Input: part model. Units: mm. Frame: model coordinates. Face numbers are marked on the shaded views. A direction names the side the tool comes from. Coordinates: 2 decimals unless noted, no trailing zeros. Write each loop counter-clockwise with the first axis right and the second up, starting at its lowest first coordinate (ties: lowest second). Pieces come first, ordered by that corner, then holes. Notation, with made-up numbers: (31, -22.75) - (50, -22.75) arc R12 cw to (50, -8.75) - close; hole circle Ø9 at (-15.5, -35.75). An arc over 180 degrees is marked (long way). Use CSV: the item, a comma, the result in double quotes.
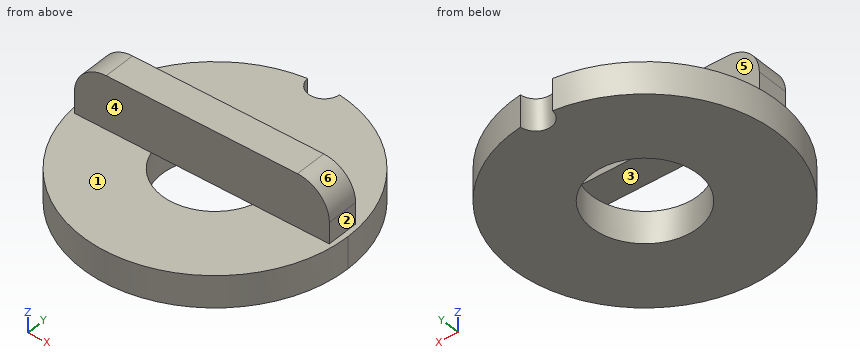
```python
from build123d import *

# Parameters (mm, degrees)
F1_DEPTH = 3
F2_W     = 24
F2_H     = 3
F3_DEPTH = 5
F4_R     = 5
F5_DEPTH = 3
F6_R     = 3


with BuildPart() as f1:
    # F0 (on Top) → F1 (new body)
    with BuildSketch(Plane.XY):
        with BuildLine():
            ThreePointArc((-1.497298, 12.41), (-8.29258, -9.353241), (12.5, 0))
            ThreePointArc((12.5, 0), (9.353241, 8.29258), (1.497298, 12.41))
            ThreePointArc((1.497298, 12.41), (0, 11), (-1.497298, 12.41))
        make_face()
    extrude(amount=F1_DEPTH)

    # F2 (on face) → F3 (join)
    with BuildSketch(Plane.XY.offset(3)):
        Rectangle(F2_W, F2_H)
    extrude(amount=F3_DEPTH)

    # F4 (on face) → F5 (cut)
    with BuildSketch(Plane(origin=(0, 0, 0), x_dir=(1, 0, 0), z_dir=(0, 0, -1))):
        Circle(F4_R)
    extrude(amount=-F5_DEPTH, mode=Mode.SUBTRACT)

    # F6
    f6_edges = [f1.edges().sort_by_distance(p)[0] for p in [
        (12, 0, 8),
        (-12, 0, 8),
    ]]
    fillet(f6_edges, radius=F6_R)


solid = f1.part
```
(1) Ray query, probe 1 along Y at (x, z) = (0, 0.9); probe 2 along Y at (x, z) = (-10.5, 6); probe 3 along Z at (x, y) = (-5, 11). Return the intervals inside material, ascending. Write a range as from..to.
Check values:
probe 1,"-12.5..-5, 5..11"
probe 2,"-1.5..1.5"
probe 3,"0..3"
(2) Reachability of the marked faces 4, 5 and 6 from +Z, -Z, +X, -X, +Y, -Y: full face, straight path, thin tool, end or side. Return the list, or none.
Check values:
face 4,"+Z, +X, -X, -Y"
face 5,"+Z, +X, -X, +Y"
face 6,"+Z, +X, +Y, -Y"
(3) Cut plane A-A on y = -3.25. Return loops of the section in (x, z).
Check values:
outline,"(-12.07, 0) - (-3.8, 0) - (-3.8, 3) - (-12.07, 3) - close; (3.8, 0) - (12.07, 0) - (12.07, 3) - (3.8, 3) - close"
(4) Pin query (flat end, axial travel): pin 1 Ø8 at (x, y) = (-4, -8.5) entering from +Z; pin 2 Ø3 at (x, z) = (-6.5, 6.5) entering from -Y; pin 3 Ø0.6 at (y, z) = (0, 4) entering from -X. Return the tip coordinate at first contact, or that it passes through.
Check values:
pin 1,"z = 3"
pin 2,"y = -1.5"
pin 3,"x = -12"
(5) Cut plane C-C on z = 0.5. Return loops of the section in (x, y).
Check values:
outline,"(-1.5, 12.41) arc R12.5 ccw (long way) to (1.5, 12.41) arc R1.5 cw to start; hole circle Ø10 at (0, 0)"
(6) Draft query along X for the marked faces 1, 2 and 3. Return one class per face: pulls with the +X half, pulls with the -X half, needs draft (parallel to the pull), parting line crosses it, or undercut.
Check values:
face 1,"needs draft"
face 2,"pulls with the +X half"
face 3,"undercut"
(7) Cut plane B-B on x = 0. Return loops of the section in (y, z), and give its area (3 significant figures).
Check values:
outline,"(-12.5, 0) - (-5, 0) - (-5, 3) - (-12.5, 3) - close; (-1.5, 3) - (1.5, 3) - (1.5, 8) - (-1.5, 8) - close; (5, 0) - (11, 0) - (11, 3) - (5, 3) - close"
area,"55.5 mm^2"
(8) Cut plane D-D on x = -7. Return loops of the section in (y, z).
Check values:
outline,"(-10.36, 0) - (10.36, 0) - (10.36, 3) - (1.5, 3) - (1.5, 8) - (-1.5, 8) - (-1.5, 3) - (-10.36, 3) - close"
